```python
from build123d import *

# Parameters (mm, degrees)
F1_DEPTH = 50.8
F2_T     = -12.7
F3_R     = 139.7
F4_DEPTH = 63.5
F7_DEPTH = 25.4


# Not quite as in the source:
# - a fillet or chamfer that OpenCascade refuses, or shapes differently, is made with other operations: its cross-section is extruded or revolved along the edge and cut away or added


with BuildPart() as f1:
    # F0 (on Top) → F1 (new body)
    with BuildSketch(Plane.XY):
        with BuildLine():
            Line((152.4, -1016), (152.4, 0))
            ThreePointArc((152.4, 0), (0, -152.4), (-152.4, 0))
            Line((-152.4, 0), (-152.4, -1016))
            Line((-152.4, -1016), (152.4, -1016))
        make_face()
        with BuildLine():
            ThreePointArc((-152.4, 0), (0, -152.4), (152.4, 0))
            Line((152.4, 0), (-152.4, 0))
        make_face()
        with BuildLine():
            Line((-152.4, 0), (152.4, 0))
            ThreePointArc((152.4, 0), (0, 152.4), (-152.4, 0))
        make_face()
    extrude(amount=F1_DEPTH)

    # F2
    f2_openings = [f1.faces().sort_by_distance(p)[0] for p in [
        (0, -447.64327, 50.8),
    ]]
    offset(amount=F2_T, openings=f2_openings)

    # F3 (on face) → F4 (join)
    with BuildSketch(Plane.XY.offset(12.7)):
        Circle(F3_R)
        with BuildLine():
            ThreePointArc((-139.7, 0), (0, -139.7), (139.7, 0))
            ThreePointArc((139.7, 0), (0, 139.7), (-139.7, 0))
        make_face()
    extrude(amount=F4_DEPTH)

    # F5: fillet of radius 12.7 on 1 edges, made by hand

    # F5_s1 → F5_t2 (revolve, cut)
    with BuildSketch(Plane.XZ):
        with BuildLine():
            ThreePointArc((-139.7, 63.5), (-135.9802561211, 72.4802561211), (-127, 76.2))
            Line((-127, 76.2), (-139.7, 76.2))
            Line((-139.7, 76.2), (-139.7, 63.5))
        make_face()
    revolve(axis=Axis((0, 0, 76.2), (0, 0, 1)), mode=Mode.SUBTRACT)

    # F6 (on face) → F7 (join)
    with BuildSketch(Plane(origin=(-152.4, 0, 0), x_dir=(0, -1, 0), z_dir=(-1, 0, 0))):
        Polygon((621.9508647919, 0), (521.6426849365, 0), (553.3189177513, -42.8551286459), (593.4422016144, -42.8551286459), align=None)
    extrude(amount=-F7_DEPTH)

    # F8: F1 across plane


with BuildPart() as f1_1:
    add(f1.part)
    add(f1.part.mirror(Plane.YZ))


solid = f1_1.part
```
Here's how the part is built. I have some questions about the finished solid (model axes, mm). A direction names the side the tool comes from. Coordinates: 2 decimals unless noted, no trailing zeros. Loops run counter-clockwise (first coordinate to the right, second up) from the corner with the lowest first, then second, coordinate; pieces in that order, holes last. Notation, with made-up numbers: (32.5, -18) - (71.5, -18) arc R6 ccw to (71.5, -7) - close; hole circle Ø3 at (85.5, 36). An arc over 180 degrees is marked (long way). Return JSON: item names as keys, results as strings. Group by question number.
Item 1: On a 3-axis mill with a long thin cutter (end or side, diameter ignored), from which of +Z, -Z, +X, -X, +Y, -Y can I reach the whole of each face in a straight line? I mean faces 4 (the face through (-127, -571, -16)), 5 (the face through (-2, -1016, 25)), 6 (the face through (-2, -495, 12.7)). Say none if no direction works.
Item 2: If we section it at C-C on x = 0: Write out the boundary of the cut face in (y, z), and give its area (3 significant figures).
Item 3: Will these pins go through, and if not, where does the flat tip stop? P1, Ø1.5, axis at x = 21.5, y = -442, coming from the +Z side; P2, Ø12, axis at x = 9.5, z = 40.5, coming from the +Y side; P3, Ø12, axis at x = 112, z = 57, coming from the +Y side (3 decimals).
Item 4: We'd pull the mould along X, two halves only. Please class faces 1 (the face through (-152.4, -501, 24)), 2 (the face through (3.351, 152.363, 25.044)), 3 (the face through (-2, -1003.3, 31)): +X half, -X half, draft (parallel to the pull), parting line (faces both ways), or undercut.
Item 5: If we section it at A-A on z = 26.5: Write out the boundary of the cut face in (x, y).
Item 6: I need wall thicknesses on line 1 (X direction, y = -852.5, z = 29); line 2 (Z direction, x = 71.5, y = -44); line 3 (Z direction, x = -137.5, y = -890). Which ranges of each line are inside material? Lowest first, please. Write a range as from..to.
Item 7: If we section it at B-B on y = -729: Write out the boundary of the cut face in (x, z).
Calculated:
{
 "1": {"face 4": "-Z, +Y, -Y", "face 5": "+Z, -Z, +X, -X, -Y", "face 6": "+Z"},
 "2": {"outline": "(-1016, 0) - (152.4, 0) - (152.4, 50.8) - (139.7, 50.8) - (139.7, 63.5) arc R12.7 ccw to (127, 76.2) - (-127, 76.2) arc R12.7 ccw to (-139.7, 63.5) - (-139.7, 12.7) - (-1003.3, 12.7) - (-1003.3, 50.8) - (-1016, 50.8) - close", "area": "33,500 mm^2"},
 "3": {"P1": "stops at z = 12.7", "P2": "stops at y = 152.36", "P3": "stops at y = 90.995"},
 "4": {"face 1": "-X half", "face 2": "parting line", "face 3": "undercut"},
 "5": {"outline": "(-152.4, -1016) - (152.4, -1016) - (152.4, 0) arc R152.4 ccw to (-152.4, 0) - close; hole (-139.7, -1003.3) - (139.7, -1003.3) - (139.7, 0) arc R139.7 cw to (-139.7, 0) - close"},
 "6": {"line 1": "x = -152.4..-139.7, 139.7..152.4", "line 2": "z = 0..76.2", "line 3": "z = 0..12.7"},
 "7": {"outline": "(-152.4, 0) - (152.4, 0) - (152.4, 50.8) - (139.7, 50.8) - (139.7, 12.7) - (-139.7, 12.7) - (-139.7, 50.8) - (-152.4, 50.8) - close"}
}
